Autodesk Inventor part; units mm, degrees
ref_plane "Work Plane1" through (12.8792, 0, 0) normal (0, 0, 1) x (-1, 0, 0)
ref_plane "YZ Plane" through (0, 0, 0) normal (1, 0, 0) x (0, 1, 0)
ref_plane "XZ Plane" through (0, 0, 0) normal (0, 1, 0) x (-1, 0, 0)
sketch "Sketch1" plane through (0, 0, 0) normal (1, 0, 0) x (0, 1, 0)
  line L0 (-4.5827, 0) -> (-2.2914, 3.9687)
  line L1 (-2.2914, 3.9687) -> (2.2914, 3.9688)
  line L2 (2.2914, 3.9688) -> (4.5827, 0)
  line L3 (4.5827, 0) -> (2.2914, -3.9687)
  line L4 (2.2914, -3.9687) -> (-2.2914, -3.9688)
  line L5 (-2.2914, -3.9688) -> (-4.5827, 0)
  point P0 (0, 0)
  point P1 (0, 0)
  dimension "d0" = 9.1654
extrude "Body" add sketch "Sketch1" along normal blind 4.3434
sketch "Sketch2" plane through (0, 0, 0) normal (-1, 0, 0) x (0, 0, 1)
  line L0 (0, -6.4158) -> (0, 6.4158)
  line L1 (-5.5563, 0) -> (5.5563, 0)
  point P0 (0, 0)
hole "Thread" at (0, 0, 0) direction (1, 0, 0) diameter 2.6416 end through all
chamfer "Chamfer1" distance 0.4296 angle 30 1 edges at (0, 0, -1.3208) measured on face at (0, -2.6537, -1.573)
chamfer "Chamfer2" distance 0.4296 angle 30 1 edges at (4.3434, 0, -1.3208) measured on face at (4.3434, -2.6537, -1.573)
sketch "Sketch3" plane through (0, 0, 0) normal (0, 0, 1) x (1, 0, 0)
  line L0 (0, 2.2914) -> (0, 4.5827)
  line L1 (0, 4.5827) -> (4.3434, 4.5827)
  line L2 (4.3434, 2.2914) -> (4.3434, 4.5827)
  line L3 (-0.8687, 0) -> (5.2121, 0)
  line L4 (0.3545, 4.5827) -> (0, 3.9688)
  line L5 (4.3434, 3.3734) -> (3.9995, 3.3734)
  line L6 (3.9995, 3.3734) -> (1.905, 4.5827)
  dimension "d3" = 30
  dimension "d5" = 7.9375
  dimension "d6" = 6.7469
  dimension "d8" = 60
  dimension "d9" = 1.905
revolve "Chamfer3" cut sketch "Sketch3" angle 360 about axis through (-10, 0, 0) along (1, 0, 0)
ref_plane "Work Plane1" through (12.8792, 0, 0) normal (0, 0, 1) x (-1, 0, 0)
equation "\"d0\" = 1.1547 * SW"
equation "\"d1\" = KOH"
equation "\"d3\" = ANG1"
equation "\"d5\" = SW0"
equation "\"d6\" = SW1"
equation "\"d8\" = ANG2"
equation "\"d9\" = KOH1"
equation "\"d10\" = -0.5 * GD1 + 0.5 * NND"
equation "\"d39\" = -0.5 * GD1 + 0.5 * NND"
equation "\"d12\" = -0.5 * GD1 + 0.5 * NND"
equation "\"d40\" = -0.5 * GD1 + 0.5 * NND"
equation "\"ANG1\" = 30deg"
equation "\"ANG2\" = 60deg"
equation "\"NND\" = 3.5052"
equation "\"KOH\" = 4.3434"
equation "\"SW\" = 7.9375"
equation "\"SW0\" = SW"
equation "\"SW1\" = 0.85 * SW"
equation "\"KOH1\" = 1.905"
equation "\"THREADDIA\" = 3.5052"
equation "\"TOA\" = 30deg"
equation "\"E0\" = 1.155 * SW"
properties part number "IFI 100/107 - No. 6 - 32 Metal Type" material "Steel, Mild"
Build history of the part. All positions in model axes, mm. A direction names the side the tool comes from. Coordinates: 2 decimals unless noted, no trailing zeros. Order: outer loops, then holes, each group sorted by start corner. A loop starts at its lowest first (then second) coordinate and runs counter-clockwise, first axis right, second up. Notation, with made-up numbers: (-29, 62) -> (10, 62) arc R21 cw to (10, 100) -> close; hole circle Ø4 at (-18.5, -22.5). An arc over 180 degrees is marked (long way). One line per item, written item: value.
(1) Slice it at A-A, the plane x = 0.85. List the corners of the cut face in (y, z).
Checked values:
outline: (-4.58, 0) -> (-2.29, -3.97) -> (2.29, -3.97) -> (4.58, 0) -> (2.29, 3.97) -> (-2.29, 3.97) -> close; hole circle Ø2.64 at (0, 0)
(2) Probe line 1 (Z direction, x = 2.2, y = 0); line 2 (Y direction, x = 1, z = 1); line 3 (Y direction, x = 2.2, z = 0). List the from-to ranges inside material, lowest first. Write a range as [from, to].
Checked values:
line 1: [-3.97, -1.32], [1.32, 3.97]
line 2: [-4.01, -0.86], [0.86, 4.01]
line 3: [-4.41, -1.32], [1.32, 4.41]
(3) Drop flat-ended pins along their axis: pin 1 Ø4 at (y, z) = (3, 2) entering from +X; pin 2 Ø1.5 at (x, z) = (3.5, 0.5) entering from +Y. Give the stop position or say it passes through.
Checked values:
pin 1: x = 4.34
pin 2: y = 4.07
(4) Slice it at B-B, the plane x = 3.1. List the corners of the cut face in (y, z), plus the area to 3 significant figures.
Checked values:
outline: circle Ø7.79 at (0, 0); hole circle Ø2.64 at (0, 0)
area: 42.1 mm2
(5) Tool access for faces 1 (the conical face through (0.11, 2.09, 3.6)), 2 (the cylindrical face through (4.169, -0.439, -3.345)): list every direction of +Z, -Z, +X, -X, +Y, -Y with a clear straight run to the whole face (end or side of a thin tool).
Checked values:
face 1: +Z, -X, +Y
face 2: +X
